Could you check a few things on this model? Use its own coordinates, in mm. A direction names the side the tool comes from. Round coordinates to 2 decimals unless told otherwise and drop trailing zeros. Loops run counter-clockwise (first coordinate to the right, second up) from the corner with the lowest first, then second, coordinate; pieces in that order, holes last. Notation, with made-up numbers: M 24,31.5 L 39,31.5 A20 cw 39,55.5 Z; hole C 16.25,18.5 d9. An arc over 180 degrees is marked long. Answer in a Markdown table with one row per item.
```python
from build123d import *

# Parameters (mm, degrees)
BOSS_EXTRUDE1_DEPTH = 12.7
SKETCH2_R           = 2.5796875
CUT_EXTRUDE1_DEPTH  = 26.162
SKETCH3_R           = 2.5796875
CUT_EXTRUDE2_DEPTH  = 26.162
FILLET1_R           = 6.35
FILLET2_R           = 6.35


with BuildPart() as part:
    # Sketch1 → Boss-Extrude1 (new body)
    with BuildSketch(Plane.XY):
        Polygon((27.808756526, 8.005672944), (6.535236668, 8.005672944), (-10.675402427, 20.509934181), (-18.140275131, 10.235418352), (2.408756526, -4.694327056), (27.808756526, -4.694327056), align=None)
    extrude(amount=BOSS_EXTRUDE1_DEPTH)

    # Sketch2 → Cut-Extrude1 (cut)
    with BuildSketch(Plane(origin=(0, 8.005672944, 0), x_dir=(1, 0, 0), z_dir=(0, 1, 0))):
        with Locations(Location((18.918756526, -6.35, 0), (0, 0, 180))):
            Circle(SKETCH2_R)
    extrude(amount=-CUT_EXTRUDE1_DEPTH, mode=Mode.SUBTRACT)

    # Sketch3 → Cut-Extrude2 (cut)
    with BuildSketch(Plane(origin=(6.064792448, 8.347470677, 0), x_dir=(0.809016994374947, -0.5877852522924737, 0), z_dir=(0.5877852522924737, 0.809016994374947, 0))):
        with Locations(Location((-11.802018822, -6.35, 0), (0, 0, 180))):
            Circle(SKETCH3_R)
    extrude(amount=-CUT_EXTRUDE2_DEPTH, mode=Mode.SUBTRACT)

    # Fillet1
    fillet1_edges = [part.edges().sort_by_distance(p)[0] for p in [
        (-14.407838779, 15.372676266, 0),
        (-14.407838779, 15.372676266, 12.7),
        (27.808756526, 1.655672944, 0),
        (27.808756526, 1.655672944, 12.7),
    ]]
    fillet(fillet1_edges, radius=FILLET1_R - 0.0001)  # a hair under: the kernel refuses the full size

    # Fillet2
    fillet2_edges = [part.edges().sort_by_distance(p)[0] for p in [
        (2.408756526, -4.694327056, 6.35),
        (6.535236668, 8.005672944, 6.35),
    ]]
    fillet(fillet2_edges, radius=FILLET2_R)


solid = part.part
```
1) Will these pins go through, and if not, where does the flat tip stop? P1, Ø4, axis at x = 7.5, z = 10.5, coming from the +Y side; P2, Ø3, axis at y = -1.5, z = 3, coming from the +X side.
Computed:
| item | result |
|---|---|
| P1 | stops at y = 8.81 |
| P2 | stops at x = 27.53 |
2) I want a section at C-C, the plane z = 11. Please give me the cut outline in (x, y), plus the area to 3 significant figures.
Computed:
| item | result |
|---|---|
| outline | M -16.5,9.04 L 0.74,-3.48 A6.35 ccw 4.47,-4.69 L 25.78,-4.69 L 25.78,8.01 L 8.6,8.01 A6.35 cw 4.87,9.22 L -9.04,19.32 Z |
| area | 541 mm² |
3) I want a section at A-A, the plane z = 8. Please give me the cut outline in (x, y), plus the area to 3 significant figures.
Computed:
| item | result |
|---|---|
| outline | M -17.96,10.11 L -12.55,6.18 L -5.09,16.45 L -10.5,20.38 Z; M -9.34,3.84 L 0.74,-3.48 A6.35 ccw 4.47,-4.69 L 16.94,-4.69 L 16.94,8.01 L 8.6,8.01 A6.35 cw 4.87,9.22 L -1.88,14.12 Z; M 20.9,-4.69 L 27.59,-4.69 L 27.59,8.01 L 20.9,8.01 Z |
| area | 486 mm² |
4) Which directions (+Z, -Z, +X, -X, +Y, -Y) give clear straight access to the entire face, cutting with the end or side of a thin tool? Please do faces 1 (the face through (2.536, -4.392, 6.439)), 2 (the face through (16, 8.006, 6)).
Computed:
| item | result |
|---|---|
| face 1 | +Z, -Z, -X, -Y |
| face 2 | +Z, -Z, +X, +Y |
5) If we mould it in two halves opening along Y, with no side actions, what happens to faces 3 (the face through (26, 1.74, 10.79)), 4 (the face through (-6.71, 9.89, 3.83)), 5 (the face through (-1.07, 13.53, 6.26)), 6 (the face through (-8.83, 3.47, 7.67))? For each: released by +Y, released by -Y, zero draft, split by the parting line, or undercut.
Computed:
| item | result |
|---|---|
| face 3 | zero draft |
| face 4 | undercut |
| face 5 | released by +Y |
| face 6 | released by -Y |
6) I want a section at D-D, the plane x = 14. Please give me the cut outline in (y, z), plus the area to 3 significant figures.
Computed:
| item | result |
|---|---|
| outline | M -4.69,0 L 8.01,0 L 8.01,12.7 L -4.69,12.7 Z |
| area | 161 mm² |
7) I need wall thicknesses on line 1 (Y direction, x = 23, z = 3); line 2 (Z direction, x = 19, y = 4); line 3 (Y direction, x = -8, z = 4.5). Which ranges of each line are inside material? Lowest first, please.
Computed:
| item | result |
|---|---|
| line 1 | y = -4.69 to 8.01 |
| line 2 | z = 0 to 3.77, 8.93 to 12.7 |
| line 3 | y = 2.87 to 6.01, 12.13 to 18.57 |
